The listing builds one solid part. Answer for the finished solid, in the listing's coordinates (mm). Face numbers are marked on the shaded views. A direction names the side the tool comes from. Coordinates: 2 decimals unless noted, no trailing zeros. Loops run counter-clockwise (first coordinate to the right, second up) from the corner with the lowest first, then second, coordinate; pieces in that order, holes last. Notation, with made-up numbers: (57.5, 69) - (115.5, 69) arc R11 ccw to (115.5, 84) - close; hole circle Ø5 at (44, 4.25). An arc over 180 degrees is marked (long way). One line per question, with ' | ' between items.
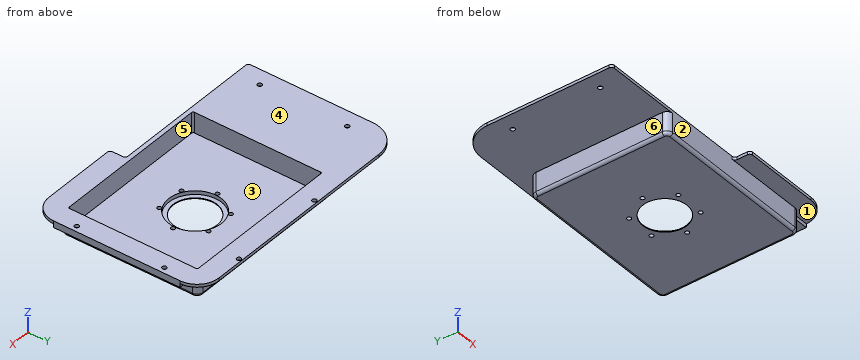
Autodesk Inventor part; units mm, degrees
ref_plane "YZ Plane" through (0, 0, 0) normal (1, 0, 0) x (0, 1, 0)
ref_plane "XZ Plane" through (0, 0, 0) normal (0, 1, 0) x (-1, 0, 0)
ref_plane "XY Plane" through (0, 0, 0) normal (0, 0, 1) x (1, 0, 0)
sketch "Sketch1" plane through (0, 0, 0) normal (0, 0, 1) x (1, 0, 0)
  line L0 (53.5, -12.0505) -> (-53.5, -12.0505)
  line L1 (-57.5, -8.0505) -> (-57.5, 78.4495)
  line L2 (-53.5, 82.4495) -> (53.5, 82.4495)
  line L3 (57.5, 78.4495) -> (57.5, -8.0505)
  line L4 (57.5, -12.0505) -> (-57.5, 82.4495) construction
  line L5 (-57.5, -12.0505) -> (57.5, 82.4495) construction
  arc A0 (-53.5, 82.4495) -> (-57.5, 78.4495) centre (-53.5, 78.4495) ccw
  arc A1 (57.5, 78.4495) -> (53.5, 82.4495) centre (53.5, 78.4495) ccw
  arc A2 (53.5, -12.0505) -> (57.5, -8.0505) centre (53.5, -8.0505) ccw
  arc A3 (-57.5, -8.0505) -> (-53.5, -12.0505) centre (-53.5, -8.0505) ccw
  point P0 (0, 0)
  point P1 (0, 35.1995)
  dimension "d0" = 115
  dimension "d1" = 94.5
  dimension "d2" = 4
extrude "Extrusion1" add sketch "Sketch1" along normal blind 15
sketch "Sketch2" plane through (0, 0, 15) normal (0, 0, 1) x (1, 0, 0)
  line L0 (53.5, 82.4495) -> (-53.5, 82.4495)
  arc A0 (-53.5, 82.4495) -> (-57.5, 78.4495) centre (-53.5, 78.4495) ccw
  line L1 (-57.5, 78.4495) -> (-57.5, -8.0505)
  arc A1 (-57.5, -8.0505) -> (-53.5, -12.0505) centre (-53.5, -8.0505) ccw
  line L2 (-53.5, -12.0505) -> (53.5, -12.0505)
  arc A2 (53.5, -12.0505) -> (57.5, -8.0505) centre (53.5, -8.0505) ccw
  line L3 (57.5, -8.0505) -> (57.5, 78.4495)
  arc A3 (57.5, 78.4495) -> (53.5, 82.4495) centre (53.5, 78.4495) ccw
  line L4 (-53.5, 93.4495) -> (53.5, 93.4495)
  arc A4 (68.5, 78.4495) -> (53.5, 93.4495) centre (53.5, 78.4495) ccw
  line L5 (68.5, 78.4495) -> (68.5, -8.0505)
  arc A5 (53.5, -23.0505) -> (68.5, -8.0505) centre (53.5, -8.0505) ccw
  line L6 (53.5, -23.0505) -> (-53.5, -23.0505)
  arc A6 (-68.5, -8.0505) -> (-53.5, -23.0505) centre (-53.5, -8.0505) ccw
  line L7 (-68.5, -8.0505) -> (-68.5, 78.4495)
  arc A7 (-53.5, 93.4495) -> (-68.5, 78.4495) centre (-53.5, 78.4495) ccw
  circle A8 centre (-32.5, 91.4495) radius 1.5
  circle A9 centre (33.5, 91.4495) radius 1.5
  circle A10 centre (64.5, 64.6495) radius 1.5
  circle A11 centre (64.5, 4.6495) radius 1.5
  point P0 (0, 0)
  dimension "d5" = 11
  dimension "d6" = 3
  dimension "d7" = 3
  dimension "d8" = 3
  dimension "d9" = 3
  dimension "d10" = 24
  dimension "d11" = 66
  dimension "d12" = 9
  dimension "d13" = 7
  dimension "d14" = 7
  dimension "d15" = 17.8
  dimension "d16" = 60
extrude "Extrusion2" add sketch "Sketch2" along normal blind 2 contours A3 L3 A2 L2 A1 L1 A0 L0 | L4 A4 L5 A5 L6 A6 L7 A7
sketch "Sketch3" plane through (0, 0, 15) normal (0, 0, -1) x (-1, 0, 0)
  circle A0 centre (-64.5, 4.6495) radius 1.5
  circle A1 centre (-64.5, 64.6495) radius 1.5
  circle A2 centre (-33.5, 91.4495) radius 1.5
  circle A3 centre (32.5, 91.4495) radius 1.5
  line L0 (53.5, -23.0505) -> (-53.5, -23.0505)
  arc A4 (53.5, -23.0505) -> (68.5, -8.0505) centre (53.5, -8.0505) ccw
  line L1 (68.5, 78.4495) -> (68.5, -8.0505)
  arc A5 (68.5, 78.4495) -> (53.5, 93.4495) centre (53.5, 78.4495) ccw
  line L2 (-53.5, 93.4495) -> (53.5, 93.4495)
  arc A6 (-53.5, 93.4495) -> (-68.5, 78.4495) centre (-53.5, 78.4495) ccw
  line L3 (-68.5, -8.0505) -> (-68.5, 78.4495)
  arc A7 (-68.5, -8.0505) -> (-53.5, -23.0505) centre (-53.5, -8.0505) ccw
  arc A8 (-53.5, 82.4495) -> (-57.5, 78.4495) centre (-53.5, 78.4495) ccw
  line L4 (-53.5, 82.4495) -> (53.5, 82.4495)
  arc A9 (57.5, 78.4495) -> (53.5, 82.4495) centre (53.5, 78.4495) ccw
  line L5 (57.5, 78.4495) -> (57.5, -8.0505)
  arc A10 (53.5, -12.0505) -> (57.5, -8.0505) centre (53.5, -8.0505) ccw
  line L6 (53.5, -12.0505) -> (-53.5, -12.0505)
  arc A11 (-57.5, -8.0505) -> (-53.5, -12.0505) centre (-53.5, -8.0505) ccw
  line L7 (-57.5, -8.0505) -> (-57.5, 78.4495)
  arc A12 (-53.5, 93.4495) -> (-68.5, 78.4495) centre (-53.5, 78.4495) ccw
  line L8 (-57.5, -8.0505) -> (-57.5, 78.4495)
  line L9 (-68.5, 78.4495) -> (-57.5, 78.4495)
  line L10 (-57.5, 78.4495) -> (-57.5, -8.0505)
  line L11 (-57.5, -8.0505) -> (-68.5, -8.0505)
  line L12 (-68.5, -8.0505) -> (-68.5, 78.4495)
  point P0 (0, 0)
  point P1 (-68.5, -0.3835)
extrude "Extrusion3" add sketch "Sketch3" along normal blind 2.5 contours L3 L9 L7 L11
sketch "Sketch4" plane through (0, 0, 17) normal (0, 0, 1) x (1, 0, 0)
  line L0 (53.5, 82.4495) -> (-53.5, 82.4495)
  arc A0 (57.5, 78.4495) -> (53.5, 82.4495) centre (53.5, 78.4495) ccw
  line L1 (57.5, -8.0505) -> (57.5, 78.4495)
  arc A1 (53.5, -12.0505) -> (57.5, -8.0505) centre (53.5, -8.0505) ccw
  line L2 (-53.5, -12.0505) -> (53.5, -12.0505)
  arc A2 (-57.5, -8.0505) -> (-53.5, -12.0505) centre (-53.5, -8.0505) ccw
  line L3 (-57.5, 78.4495) -> (-57.5, -8.0505)
  arc A3 (-53.5, 82.4495) -> (-57.5, 78.4495) centre (-53.5, 78.4495) ccw
  line L4 (-53.5, 79.4495) -> (53.5, 79.4495)
  arc A4 (54.5, 78.4495) -> (53.5, 79.4495) centre (53.5, 78.4495) ccw
  line L5 (54.5, 78.4495) -> (54.5, -8.0505)
  arc A5 (53.5, -9.0505) -> (54.5, -8.0505) centre (53.5, -8.0505) ccw
  line L6 (53.5, -9.0505) -> (-53.5, -9.0505)
  arc A6 (-54.5, -8.0505) -> (-53.5, -9.0505) centre (-53.5, -8.0505) ccw
  line L7 (-54.5, -8.0505) -> (-54.5, 78.4495)
  arc A7 (-53.5, 79.4495) -> (-54.5, 78.4495) centre (-53.5, 78.4495) ccw
  point P0 (0, 0)
  dimension "d21" = 3
extrude "Extrusion4" cut sketch "Sketch4" against normal blind 14 contours L4 A4 L5 A5 L6 A6 L7 A7
sketch "Sketch7" plane through (0, 0, 17) normal (0, 0, 1) x (1, 0, 0)
  arc A0 (53.5, -9.0505) -> (54.5, -8.0505) centre (53.5, -8.0505) ccw
  line L0 (53.5, -9.0505) -> (-53.5, -9.0505)
  arc A1 (-54.5, -8.0505) -> (-53.5, -9.0505) centre (-53.5, -8.0505) ccw
  line L1 (-54.5, -8.0505) -> (-54.5, 78.4495)
  arc A2 (-53.5, 79.4495) -> (-54.5, 78.4495) centre (-53.5, 78.4495) ccw
  line L2 (-53.5, 79.4495) -> (53.5, 79.4495)
  arc A3 (54.5, 78.4495) -> (53.5, 79.4495) centre (53.5, 78.4495) ccw
  line L3 (54.5, 78.4495) -> (54.5, -8.0505)
  line L4 (-53.5, -23.0505) -> (53.5, -23.0505)
  arc A4 (53.5, -23.0505) -> (68.5, -8.0505) centre (53.5, -8.0505) ccw
  line L5 (68.5, -8.0505) -> (68.5, 78.4495)
  arc A5 (68.5, 78.4495) -> (53.5, 93.4495) centre (53.5, 78.4495) ccw
  line L6 (53.5, 93.4495) -> (-53.5, 93.4495)
  arc A6 (-53.5, 93.4495) -> (-68.5, 78.4495) centre (-53.5, 78.4495) ccw
  line L7 (-68.5, 78.4495) -> (-68.5, -8.0505)
  arc A7 (-68.5, -8.0505) -> (-53.5, -23.0505) centre (-53.5, -8.0505) ccw
  circle A8 centre (-32.5, 91.4495) radius 1.5
  circle A9 centre (33.5, 91.4495) radius 1.5
  circle A10 centre (64.5, 64.6495) radius 1.5
  circle A11 centre (64.5, 4.6495) radius 1.5
  line L8 (-53.5, -12.0505) -> (53.5, -12.0505)
  line L9 (-75.3145, -26.4449) -> (0.399, -26.4449)
  line L10 (0.399, -26.4449) -> (0.399, -12.0505)
  line L11 (0.399, -12.0505) -> (-75.3145, -12.0505)
  line L12 (-75.3145, -12.0505) -> (-75.3145, -26.4449)
  point P0 (0, 0)
extrude "Extrusion7" cut sketch "Sketch7" against normal through all contours A7 L11 L8 L10 L4 | L4 L10 L9 L12 L11 A7
fillet "Fillet1" radius 2 10 edges at (56.3284, -10.8789, 0) (57.5, 35.1995, 0) (56.3284, 81.2779, 0) (0, 82.4495, 0) (-56.3284, 81.2779, 0) (-57.5, 35.1995, 0) (-56.3284, -10.8789, 0) (0, -12.0505, 0) (0.399, -12.0505, 16) (0.399, -23.0505, 16)
sketch "Sketch8" plane through (0, 0, 17) normal (0, 0, 1) x (1, 0, 0)
  circle A0 centre (64.5, 64.6495) radius 1.5
  circle A1 centre (64.5, 4.6495) radius 1.5
  circle A2 centre (-95.5, 64.6495) radius 1.5
  circle A3 centre (-95.5, 4.6495) radius 1.5
  arc A4 (0.399, -21.0505) -> (2.399, -23.0505) centre (2.399, -21.0505) ccw
  line L0 (2.399, -23.0505) -> (53.5, -23.0505)
  arc A5 (53.5, -23.0505) -> (68.5, -8.0505) centre (53.5, -8.0505) ccw
  line L1 (68.5, -8.0505) -> (68.5, 78.4495)
  arc A6 (68.5, 78.4495) -> (53.5, 93.4495) centre (53.5, 78.4495) ccw
  line L2 (53.5, 93.4495) -> (-53.5, 93.4495)
  arc A7 (-53.5, 93.4495) -> (-68.5, 78.4495) centre (-53.5, 78.4495) ccw
  line L3 (-68.5, 78.4495) -> (-68.5, -8.0505)
  arc A8 (-68.5, -8.0505) -> (-68.3214, -10.3582) centre (-53.5, -8.0505) ccw
  arc A9 (-68.3214, -10.3582) -> (-66.3452, -12.0505) centre (-66.3452, -10.0505) ccw
  line L4 (-66.3452, -12.0505) -> (-1.601, -12.0505)
  arc A10 (0.399, -14.0505) -> (-1.601, -12.0505) centre (-1.601, -14.0505) ccw
  line L5 (0.399, -14.0505) -> (0.399, -21.0505)
  arc A11 (53.5, -9.0505) -> (54.5, -8.0505) centre (53.5, -8.0505) ccw
  line L6 (53.5, -9.0505) -> (-53.5, -9.0505)
  arc A12 (-54.5, -8.0505) -> (-53.5, -9.0505) centre (-53.5, -8.0505) ccw
  line L7 (-54.5, -8.0505) -> (-54.5, 78.4495)
  arc A13 (-53.5, 79.4495) -> (-54.5, 78.4495) centre (-53.5, 78.4495) ccw
  line L8 (-53.5, 79.4495) -> (53.5, 79.4495)
  arc A14 (54.5, 78.4495) -> (53.5, 79.4495) centre (53.5, 78.4495) ccw
  line L9 (54.5, 78.4495) -> (54.5, -8.0505)
  circle A15 centre (-32.5, 91.4495) radius 1.5
  circle A16 centre (33.5, 91.4495) radius 1.5
  circle A17 centre (64.5, 64.6495) radius 1.5
  circle A18 centre (64.5, 4.6495) radius 1.5
  line L10 (-106.5344, -10.0505) -> (-106.5344, 73.4495)
  arc A19 (-86.5344, 93.4495) -> (-106.5344, 73.4495) centre (-86.5344, 73.4495) ccw
  line L11 (-53.5, 93.4495) -> (-86.5344, 93.4495)
  line L12 (-53.5, -12.0505) -> (-66.3452, -12.0505)
  line L13 (-66.3452, -12.0505) -> (-104.5344, -12.0505)
  arc A20 (-106.5344, -10.0505) -> (-104.5344, -12.0505) centre (-104.5344, -10.0505) ccw
  point P0 (0, 0)
  dimension "d37" = 3
  dimension "d38" = 3
  dimension "d39" = 160
  dimension "d40" = 0
  dimension "d41" = 0
  dimension "d42" = 2
  dimension "d54" = 20
extrude "Extrusion8" add sketch "Sketch8" against normal up to surface (2 mm away) contours L13 A20 L10 A19 L11 A7 L3 A8 A9
sketch "Skizze9" plane through (0, 0, 3) normal (0, 0, 1) x (1, 0, 0)
  line L0 (53.5, -9.0505) -> (-53.5, -9.0505)
  arc A0 (53.5, -9.0505) -> (54.5, -8.0505) centre (53.5, -8.0505) ccw
  line L1 (54.5, 78.4495) -> (54.5, -8.0505)
  arc A1 (54.5, 78.4495) -> (53.5, 79.4495) centre (53.5, 78.4495) ccw
  line L2 (-53.5, 79.4495) -> (53.5, 79.4495)
  arc A2 (-53.5, 79.4495) -> (-54.5, 78.4495) centre (-53.5, 78.4495) ccw
  line L3 (-54.5, -8.0505) -> (-54.5, 78.4495)
  arc A3 (-54.5, -8.0505) -> (-53.5, -9.0505) centre (-53.5, -8.0505) ccw
  circle A4 centre (0, 35.1995) radius 15
  point P0 (0, 0)
  dimension "d45" = 30
extrude "Extrusion9" cut sketch "Skizze9" against normal blind 13 contours A4
sketch "Skizze10" plane through (0, 0, 3) normal (0, 0, 1) x (1, 0, 0)
  circle A0 centre (19.4922, 35.1995) radius 4
  circle A1 centre (-9.7461, 52.0802) radius 4
  circle A2 centre (-9.7461, 18.3188) radius 4
  circle A3 centre (9.7461, 52.0802) radius 1.45
  circle A4 centre (9.7461, 18.3188) radius 1.45
  circle A5 centre (-19.4922, 35.1995) radius 1.45
  circle A6 centre (0, 35.1995) radius 13.5
  circle A7 centre (0, 35.1995) radius 23.9428
  circle A8 centre (19.4922, 35.1995) radius 1.4
  point P0 (0, 0)
  dimension "d48" = 2.8
extrude "Extrusion10" cut sketch "Skizze10" against normal blind 14 contours A8
pattern_circular "Runde Anordnung1" count 6 over 360 about axis through (0, 35.1995, 3) along (0, 0, -1) of "Extrusion10"
sketch "Skizze11" plane through (0, 0, 3) normal (0, 0, 1) x (1, 0, 0)
  circle A0 centre (9.7461, 52.0802) radius 1.4
  circle A1 centre (-9.7461, 52.0802) radius 1.4
  circle A2 centre (-19.4922, 35.1995) radius 1.4
  circle A3 centre (-9.7461, 18.3188) radius 1.4
  circle A4 centre (9.7461, 18.3188) radius 1.4
  circle A5 centre (19.4922, 35.1995) radius 1.4
  circle A6 centre (0, 35.1995) radius 15
  line L0 (53.5, -9.0505) -> (-53.5, -9.0505)
  arc A7 (53.5, -9.0505) -> (54.5, -8.0505) centre (53.5, -8.0505) ccw
  line L1 (54.5, 78.4495) -> (54.5, -8.0505)
  arc A8 (54.5, 78.4495) -> (53.5, 79.4495) centre (53.5, 78.4495) ccw
  line L2 (-53.5, 79.4495) -> (53.5, 79.4495)
  arc A9 (-53.5, 79.4495) -> (-54.5, 78.4495) centre (-53.5, 78.4495) ccw
  line L3 (-54.5, -8.0505) -> (-54.5, 78.4495)
  arc A10 (-54.5, -8.0505) -> (-53.5, -9.0505) centre (-53.5, -8.0505) ccw
  circle A11 centre (0, 35.1995) radius 18.05
  point P0 (0, 0)
  dimension "d55" = 36.1
extrude "Extrusion11" cut sketch "Skizze11" against normal blind 2.5 contours A6 | A11
properties part number "30_XYTable_Aliexpress_sampleinsert_round"
Item 1: Find section C-C, the plane y = -4. Write down the section's boundary in (x, z), plus the area to 3 significant figures.
Taken from the geometry:
outline: (-106.53, 15) - (-57.5, 15) - (-57.5, 2) arc R2 ccw to (-55.5, 0) - (55.5, 0) arc R2 ccw to (57.5, 2) - (57.5, 12.5) - (68.5, 12.5) - (68.5, 17) - (54.5, 17) - (54.5, 3) - (-54.5, 3) - (-54.5, 17) - (-106.53, 17) - close | area: 575 mm2
Item 2: The mould has two halves that part along Y. Classify the marked faces 1, 2 and 3: pulls with the +Y half, pulls with the -Y half, needs draft (parallel to the pull), parting line crosses it, or undercut.
Taken from the geometry:
face 1: needs draft | face 2: pulls with the -Y half | face 3: undercut
Item 3: Find section B-B, the plane x = -3.5. Write down the section's boundary in (y, z).
Taken from the geometry:
outline: (-12.05, 2) arc R2 ccw to (-10.05, 0) - (20.61, 0) - (20.61, 0.5) - (17.49, 0.5) - (17.49, 3) - (-9.05, 3) - (-9.05, 17) - (-12.05, 17) - close; (49.79, 0) - (80.45, 0) arc R2 ccw to (82.45, 2) - (82.45, 15) - (93.45, 15) - (93.45, 17) - (79.45, 17) - (79.45, 3) - (52.91, 3) - (52.91, 0.5) - (49.79, 0.5) - close
Item 4: Find the intervals of material crossed by line 1 (Y direction, x = -32.5, z = 15.7); line 2 (X direction, y = 23, z = 8.25); line 3 (X direction, y = 39, z = 14.75), in increasing order. Write a range as [from, to].
Taken from the geometry:
line 1: y = [-12.05, -9.05], [79.45, 89.95], [92.95, 93.45] | line 2: x = [-57.5, -54.5], [54.5, 57.5] | line 3: x = [-57.5, -54.5], [54.5, 68.5]
Item 5: Which of the six approach directions +Z, -Z, +X, -X, +Y, -Y give full straight-line access (tool end or side, diameter ignored) to the marked faces 4, 5 and 6?
Taken from the geometry:
face 4: +Z, +X, -X, +Y, -Y | face 5: +Z | face 6: -Z, -X, +Y, -Y
Item 6: Find section A-A, the plane z = 6.75. Write down the section's boundary in (x, y), plus the area to 3 significant figures.
Taken from the geometry:
outline: (-57.5, -8.05) arc R4 ccw to (-53.5, -12.05) - (53.5, -12.05) arc R4 ccw to (57.5, -8.05) - (57.5, 78.45) arc R4 ccw to (53.5, 82.45) - (-53.5, 82.45) arc R4 ccw to (-57.5, 78.45) - close; hole (-54.5, -8.05) arc R1 ccw to (-53.5, -9.05) - (53.5, -9.05) arc R1 ccw to (54.5, -8.05) - (54.5, 78.45) arc R1 ccw to (53.5, 79.45) - (-53.5, 79.45) arc R1 ccw to (-54.5, 78.45) - close | area: 1,210 mm2
Item 7: Find section D-D, the plane x = -25. Write down the section's boundary in (y, z), plus the area to 3 significant figures.
Taken from the geometry:
outline: (-12.05, 2) arc R2 ccw to (-10.05, 0) - (80.45, 0) arc R2 ccw to (82.45, 2) - (82.45, 15) - (93.45, 15) - (93.45, 17) - (79.45, 17) - (79.45, 3) - (-9.05, 3) - (-9.05, 17) - (-12.05, 17) - close | area: 388 mm2
Item 8: Each of these flat-tipped pins is pushed along its axis until it touches: pin 1 Ø6.5 at (x, z) = (25, 11) entering from +Y; pin 2 Ø6.5 at (y, z) = (20.5, 10.5) entering from -X; pin 3 Ø9 at (x, y) = (61.5, 21) entering from -Z; pin 4 Ø2.5 at (x, y) = (-32.5, 91.45) entering from -Z. Where does it stop, or does it pass through?
Taken from the geometry:
pin 1: stops at y = 82.45 | pin 2: stops at x = -57.5 | pin 3: stops at z = 0.68 | pin 4: passes through
